from build123d import *

# Parameters (mm, degrees)
F0_R     = 2.5
F1_DEPTH = 12
F0_W     = 7
F0_H     = 14
F2_DEPTH = 12.001
F3_R     = 8.075
F4_DEPTH = 64.001
F6_DEPTH = 64.001


with BuildPart() as f1:
    # F0 (on Top) → F1 (new body)
    with BuildSketch(Plane.XY):
        Polygon((-25, -32), (25, -32), (25, -18), (32, -18), (32, 18), (25, 18), (25, 32), (-25, 32), (-25, 18), (-32, 18), (-32, -18), (-25, -18), align=None)
        with Locations((-13, -27)):
            Circle(F0_R, mode=Mode.SUBTRACT)
        with Locations((-13, -13)):
            Circle(F0_R, mode=Mode.SUBTRACT)
        with Locations((13, -27)):
            Circle(F0_R, mode=Mode.SUBTRACT)
        with Locations((13, -13)):
            Circle(F0_R, mode=Mode.SUBTRACT)
        with Locations((-13, 13)):
            Circle(F0_R, mode=Mode.SUBTRACT)
        with Locations((-13, 27)):
            Circle(F0_R, mode=Mode.SUBTRACT)
        with Locations((13, 13)):
            Circle(F0_R, mode=Mode.SUBTRACT)
        with Locations((13, 27)):
            Circle(F0_R, mode=Mode.SUBTRACT)
    extrude(amount=F1_DEPTH)

    # F0 (on Top) → F2 (cut, through all)
    with BuildSketch(Plane.XY):
        with Locations((28.5, -25)):
            Rectangle(F0_W, F0_H)
        with Locations((-28.5, -25)):
            Rectangle(F0_W, F0_H)
    extrude(amount=F2_DEPTH, mode=Mode.SUBTRACT)

    # F3 (on face) → F4 (cut, through all)
    with BuildSketch(Plane.XZ.offset(32)):
        with Locations((0, 12)):
            Circle(F3_R)
    extrude(amount=-F4_DEPTH, mode=Mode.SUBTRACT)

    # F5 (on face) → F6 (cut, through all)
    with BuildSketch(Plane(origin=(-32, 0, 0), x_dir=(0, -1, 0), z_dir=(-1, 0, 0))):
        with BuildLine():
            ThreePointArc((-8.075, 12), (0, 3.925), (8.075, 12))
            Line((8.075, 12), (-8.075, 12))
        make_face()
    extrude(amount=-F6_DEPTH, mode=Mode.SUBTRACT)


solid = f1.part
Input: part model. Units: mm. Frame: model coordinates. A direction names the side the tool comes from. Coordinates: 2 decimals unless noted, no trailing zeros. Loops run counter-clockwise (first coordinate to the right, second up) from the corner with the lowest first, then second, coordinate; pieces in that order, holes last. Notation, with made-up numbers: (83, -31.5) -> (115, -31.5) arc R34 ccw to (115, 6.5) -> close; hole circle Ø7 at (-11.5, 56.5). An arc over 180 degrees is marked (long way). Write each question's results on one line, items separated by ' | '. Start each with the question number.
Q1. Pull-direction query (Y, two-part tool) for faces 1 (the flat face through (0, -32, 3)), 2 (the cylindrical face through (-0.178, 19.332, 3.927)), 3 (the cylindrical face through (11.16, -25.31, 5.92)); classes: released by +Y, released by -Y, zero draft, split by the parting line, or undercut.
Q2. Section C-C, the plane x = -13. Return the cut outline in (y, z) (3 decimals), plus the area to 3 significant figures.
Q3. Section A-A, the plane y = 27. Return the cut outline in (x, z) (3 decimals), plus the area to 3 significant figures.
Q4. Ray query, line 1 (Y direction, x = 13, z = 2.5); line 2 (Y direction, x = -13, z = 7); line 3 (X direction, y = 14, z = 2). Return the intervals inside material, ascending. Write a range as from..to.
Q5. Pin query (flat end, axial travel): pin 1 (3.5 mm diameter, centred on y = 25.5, z = 6, fed in from -X); pin 2 (2 mm diameter, centred on x = 28.5, z = 4, fed in from +Y); pin 3 (4.5 mm diameter, centred on x = -13, y = 27, fed in from -Z); pin 4 (5 mm diameter, centred on x = -2, y = -13, fed in from +Z). Return the tip coordinate at first contact, or that it passes through.
Q6. Section B-B, the plane z = 6.25. State how many separate pieces and enclosed holes the cut face has, plus the area to 3 significant figures.
Q7. Reachability of faces 4 (the flat face through (28, -18, 6)), 5 (the flat face through (-28, 18, 6)), 6 (the flat face through (-25, -25, 6)), 7 (the flat face through (25, 25, 6)) from +Z, -Z, +X, -X, +Y, -Y: full face, straight path, thin tool, end or side. Return the list, or none.
Found:
1) face 1: released by -Y | face 2: zero draft | face 3: undercut
2) outline: (-32, 0) -> (-29.5, 0) -> (-29.5, 12) -> (-32, 12) -> close; (-24.5, 0) -> (-15.5, 0) -> (-15.5, 12) -> (-24.5, 12) -> close; (-10.5, 0) -> (10.5, 0) -> (10.5, 12) -> (8.075, 12) arc R8.075 cw to (-8.075, 12) -> (-10.5, 12) -> close; (15.5, 0) -> (24.5, 0) -> (24.5, 12) -> (15.5, 12) -> close; (29.5, 0) -> (32, 0) -> (32, 12) -> (29.5, 12) -> close | area: 426 mm2
3) outline: (-25, 0) -> (-15.5, 0) -> (-15.5, 12) -> (-25, 12) -> close; (-10.5, 0) -> (10.5, 0) -> (10.5, 12) -> (8.075, 12) arc R8.075 cw to (-8.075, 12) -> (-10.5, 12) -> close; (15.5, 0) -> (25, 0) -> (25, 12) -> (15.5, 12) -> close | area: 378 mm2
4) line 1: -32..-29.5, -24.5..-15.5, -10.5..10.5, 15.5..24.5, 29.5..32 | line 2: -32..-29.5, -24.5..-15.5, -10.5..-6.34, 6.34..10.5, 15.5..24.5, 29.5..32 | line 3: -32..-15.29, -10.71..10.71, 15.29..32
5) pin 1: x = -25 | pin 2: y = 18 | pin 3: through | pin 4: z = 5.3
6) separate pieces: 4 | enclosed holes: 8 | area: 2,220 mm2
7) face 4: +Z, -Z, +X, -Y | face 5: +Z, -Z, -X, +Y | face 6: +Z, -Z, -X, -Y | face 7: +Z, -Z, +X, +Y
